from build123d import *

# Parameters (mm, degrees)
SKETCH1_R           = 5
BOSS_EXTRUDE1_DEPTH = 5


with BuildPart() as part:
    # Sketch1 → Boss-Extrude1 (new, symmetric)
    with BuildSketch(Plane(origin=(0, 0, 0), x_dir=(0, 0, -1), z_dir=(1, 0, 0))):
        with BuildLine():
            Line((0, 15), (30, 15))
            Line((30, 15), (30, -15))
            Line((30, -15), (0, -15))
            ThreePointArc((0, -15), (-15, 0), (0, 15))
        make_face()
        Circle(SKETCH1_R, mode=Mode.SUBTRACT)
    extrude(amount=BOSS_EXTRUDE1_DEPTH, both=True)

    # Sketch2 → Revolve1 (revolve)
    with BuildSketch(Plane(origin=(0, 0, 0), x_dir=(0, 0, -1), z_dir=(1, 0, 0)), mode=Mode.PRIVATE) as revolve1_sk:
        Polygon((30, 0), (30, 19.46387593), (33.500252175, 19.46387593), (33.500252175, 14.525280545), (290.484846339, 14.525280545), (290.484846339, 0), align=None)
    revolve(revolve1_sk.sketch.rotate(Axis((0, 0, -290.484846339), (0, 0, 1)), 90), axis=Axis((0, 0, -290.484846339), (0, 0, 1)))


solid = part.part
CAD build for the part. Positions are in the model's coordinates, mm. A direction names the side the tool comes from. Round coordinates to 2 decimals unless told otherwise and drop trailing zeros. Loops run counter-clockwise (first coordinate to the right, second up) from the corner with the lowest first, then second, coordinate; pieces in that order, holes last. Notation, with made-up numbers: M -8.5,17 L 14.5,17 A17 cw 14.5,41 Z; hole C 18,1.5 d10. An arc over 180 degrees is marked long. One line per question, with ' | ' between items. Start each with the question number.
Item 1: Cut at C-C, the plane z = -17. Write the cut outline in (x, y), plus the area to 3 significant figures.
Item 2: Pin check, flat tips, straight feed: pin 1 Ø5 at (y, z) = (13.5, -99) entering from -X; pin 2 Ø13 at (y, z) = (0, 0) entering from +X; pin 3 Ø9 at (y, z) = (-7, 0.5) entering from -X. Stop position of each tip, or through.
Item 3: Cut at D-D, the plane y = 11. Write the cut outline in (x, z), plus the area to 3 significant figures.
Item 4: Two-plate mould, pull along Y, no slides. Class faces 1 (the flat face through (-5, 0, -8)), 2 (the cylindrical face through (0, 0, 15)), 3 (the cylindrical face through (-0.07, -4.88, 1.08)): pulls with the +Y half, pulls with the -Y half, needs draft (parallel to the pull), parting line crosses it, or undercut.
Item 5: Cut at B-B, the plane y = 0. Write the cut outline in (x, z).
Item 6: Which spindle directions (+Z, -Z, +X, -X, +Y, -Y) get a long thin tool onto all of the face, cutting with end or side? Do faces 4 (the flat face through (15, 1, -33.5)), 5 (the flat face through (0, 15, -15)), 6 (the flat face through (0, 0, -290.485)), 7 (the flat face through (5, 0, -8)), 8 (the flat face through (0, -15, -15)). Say none if no direction does.
Item 7: Cut at A-A, the plane x = 0. Write the cut outline in (y, z).
Item 8: Wall check: line 1 (X direction, y = -12, z = -19); line 2 (Z direction, x = -13.5, y = -8); line 3 (Z direction, x = -12, y = -2.5). Give the ranges that are in metal, low to high.
Responses:
1) outline: M -5,-15 L 5,-15 L 5,15 L -5,15 Z | area: 300 mm²
2) pin 1: stops at x = -9.49 | pin 2: stops at x = 5 | pin 3: stops at x = -5
3) outline: M -16.06,-33.5 L -9.49,-33.5 L -9.49,-290.48 L 9.49,-290.48 L 9.49,-33.5 L 16.06,-33.5 L 16.06,-30 L 5,-30 L 5,10.2 L -5,10.2 L -5,-30 L -16.06,-30 Z | area: 5,390 mm²
4) face 1: needs draft | face 2: parting line crosses it | face 3: undercut
5) outline: M -19.46,-33.5 L -14.53,-33.5 L -14.53,-290.48 L 14.53,-290.48 L 14.53,-33.5 L 19.46,-33.5 L 19.46,-30 L 5,-30 L 5,-5 L -5,-5 L -5,-30 L -19.46,-30 Z; M -5,5 L 5,5 L 5,15 L -5,15 Z
6) face 4: -Z | face 5: +Z, +X, -X, +Y | face 6: -Z, +X, -X, +Y, -Y | face 7: +Z, +X, +Y, -Y | face 8: +Z, +X, -X, -Y
7) outline: M -19.46,-33.5 L -14.53,-33.5 L -14.53,-290.48 L 14.53,-290.48 L 14.53,-33.5 L 19.46,-33.5 L 19.46,-30 L 15,-30 L 15,0 A15 ccw -15,0 L -15,-30 L -19.46,-30 Z; hole C 0,0 d10
8) line 1: x = -5 to 5 | line 2: z = -33.5 to -30 | line 3: z = -290.48 to -30
